Geometry: final body of the model. Coordinates: model frame, mm. A direction names the side the tool comes from. Give positions to 0.01 mm unless a question says otherwise; leave off trailing zeros. Write each loop counter-clockwise with the first axis right and the second up, starting at its lowest first coordinate (ties: lowest second). Pieces come first, ordered by that corner, then holes.
Q1. Mould query, pull axis Z, two halves, no side actions, for faces 1 (the flat face through (30, 4, 60)), 2 (the flat face through (52, 4, 40)), 3 (the flat face through (52, 4, 20)), 4 (the flat face through (0, 4, 30)). Classes: +Z half, -Z half, draft (parallel to the pull), parting line (faces both ways), or undercut.
Q2. Reachability of faces 5 (the flat face through (52, 4, 30)), 6 (the cylindrical face through (54, 4.06, 3.69)) from +Z, -Z, +X, -X, +Y, -Y: full face, straight path, thin tool, end or side. Return the list, or none.
Q3. Line query: line 1 (X direction, y = 1.5, z = 5); line 2 (Y direction, x = 55, z = 10); line 3 (X direction, y = 5.75, z = 4). Output: solid intervals per line, ascending.
Q4. Section A-A (x = 55). Return the cut outline in (y, z).
Q5. Section B-B (z = 55). Return the cut outline in (x, y), plus the area to 3 significant figures.
Q6. Section D-D (z = 10). Return the cut outline in (x, y), plus the area to 4 significant figures.
Q7. Pin query (flat end, axial travel): pin 1 Ø2 at (y, z) = (4, 10) entering from +X; pin 2 Ø3 at (y, z) = (4, 20) entering from -X. Return the tip coordinate at first contact, or that it passes through.
Q8. Section C-C (x = 5). Return the cut outline in (y, z).
from build123d import *

# Parameters (mm, degrees)
SKETCH_1_W          = 60
SKETCH_1_H          = 60
EXTRUDE_1_DEPTH     = 8
SKETCH_2_R          = 1.65
CUT_EXTRUDE_1_DEPTH = 8
SKETCH_3_W          = 1
SKETCH_3_H          = 60
EXTRUDE_2_DEPTH     = 8
SKETCH_7_R          = 1.25
CUT_EXTRUDE_2_DEPTH = 9


with BuildPart() as part:
    # 草图1 → 凸台-拉伸1 (new body)
    with BuildSketch(Plane(origin=(0, 0, 0), x_dir=(1, 0, 0), z_dir=(0, 1, 0))):
        with Locations((30, -30)):
            Rectangle(SKETCH_1_W, SKETCH_1_H)
    extrude(amount=EXTRUDE_1_DEPTH)

    # 草图2 → 切除-拉伸1 (cut)
    with BuildSketch(Plane(origin=(0, 8, 0), x_dir=(1, 0, 0), z_dir=(0, 1, 0))):
        with Locations(Location((5, -5, 0), (0, 0, 270))):
            Circle(SKETCH_2_R)
        with Locations(Location((55, -5, 0), (0, 0, 270))):
            Circle(SKETCH_2_R)
        with Locations(Location((5, -55, 0), (0, 0, 270))):
            Circle(SKETCH_2_R)
        with Locations(Location((55, -55, 0), (0, 0, 270))):
            Circle(SKETCH_2_R)
    extrude(amount=-CUT_EXTRUDE_1_DEPTH, mode=Mode.SUBTRACT)

    # 草图3 → 凸台-拉伸2 (add)
    with BuildSketch(Plane(origin=(0, 8, 0), x_dir=(1, 0, 0), z_dir=(0, 1, 0))):
        with Locations((60.5, -30)):
            Rectangle(SKETCH_3_W, SKETCH_3_H)
    extrude(amount=-EXTRUDE_2_DEPTH)

    # 草图7 → 切除-拉伸2 (cut)
    with BuildSketch(Plane(origin=(61, 0, 0), x_dir=(0, 0, -1), z_dir=(1, 0, 0))):
        with Locations((-50, 4)):
            Circle(SKETCH_7_R)
        with Locations((-40, 4)):
            Circle(SKETCH_7_R)
        with Locations((-30, 4)):
            Circle(SKETCH_7_R)
        with Locations((-10, 4)):
            Circle(SKETCH_7_R)
        with Locations((-20, 4)):
            Circle(SKETCH_7_R)
    extrude(amount=-CUT_EXTRUDE_2_DEPTH, mode=Mode.SUBTRACT)


solid = part.part
Computed:
1. face 1: +Z half
1. face 2: undercut
1. face 3: undercut
1. face 4: draft
2. face 5: +X
2. face 6: +Y, -Y
3. line 1: x = 0 to 3.35, 6.65 to 53.35, 56.65 to 61
3. line 2: y = 0 to 2.75, 5.25 to 8
3. line 3: x = 0 to 3.69, 6.31 to 53.69, 56.31 to 61
4. outline: (0, 0) - (8, 0) - (8, 3.35) - (0, 3.35) - close; (0, 6.65) - (8, 6.65) - (8, 53.35) - (0, 53.35) - close; (0, 56.65) - (8, 56.65) - (8, 60) - (0, 60) - close; hole circle Ø2.5 at (4, 10); hole circle Ø2.5 at (4, 20); hole circle Ø2.5 at (4, 30); hole circle Ø2.5 at (4, 40); hole circle Ø2.5 at (4, 50)
5. outline: (0, 0) - (3.35, 0) - (3.35, 8) - (0, 8) - close; (6.65, 0) - (53.35, 0) - (53.35, 8) - (6.65, 8) - close; (56.65, 0) - (61, 0) - (61, 8) - (56.65, 8) - close
5. area: 435 mm2
6. outline: (0, 0) - (61, 0) - (61, 2.75) - (52, 2.75) - (52, 5.25) - (61, 5.25) - (61, 8) - (0, 8) - close
6. area: 465.5 mm2
7. pin 1: stops at x = 52
7. pin 2: stops at x = 0
8. outline: (0, 0) - (8, 0) - (8, 3.35) - (0, 3.35) - close; (0, 6.65) - (8, 6.65) - (8, 53.35) - (0, 53.35) - close; (0, 56.65) - (8, 56.65) - (8, 60) - (0, 60) - close
